Source: CAD feature listing. Evaluate the final solid. Frame: model axes, mm. A direction names the side the tool comes from. Round coordinates to 2 decimals unless told otherwise and drop trailing zeros. Order: outer loops, then holes, each group sorted by start corner. A loop starts at its lowest first (then second) coordinate and runs counter-clockwise, first axis right, second up. Notation, with made-up numbers: (73.5, -7) -> (77.5, -7) arc R18 cw to (77.5, 0) -> close; hole circle Ø3 at (-5.75, 24). An arc over 180 degrees is marked (long way). Answer as CSV lines item,"result". Start each with the question number.
(1) Section query C-C (z = 43). Output: boundary loops of the cut face in (x, y).
(2) Set-up query: faces 1 (the flat face through (17, 18, 5)), 2 (the flat face through (23.42, -21.22, 32.33)), 3 (the flat face through (0, 20, 5)), 4 (the flat face through (20, 0, 5)). Return all of +Z, -Z, +X, -X, +Y, -Y with unobstructed straight access to the full face (end or side cutting, diameter ignored); none if empty.
(3) Line query: line 1 along Y through (x, z) = (-15, 37); line 2 along X through (y, z) = (7.5, 8.5); line 3 along Z through (x, y) = (15, -24). Output: solid intervals per line, ascending. Write a range as from..to.
(4) Contact query for flat-ended pins moving along their axis: P1, Ø5, axis at x = 7, z = 4.5, coming from the +Y side; P2, Ø12, axis at y = -24.5, z = 8, coming from the +X side; P3, Ø12, axis at x = 25, z = 20, coming from the -Y side. Output: stop coordinate, or through.
(5) Section query A-A (z = 8.5). Output: boundary loops of the cut face in (x, y), plus the area to 3 significant figures.
(6) Section query B-B (z = 34.5). Output: boundary loops of the cut face in (x, y), plus the area to 3 significant figures.
(7) Pull-direction query (Z, two-part tool) for faces 5 (the flat face through (-21, -2, 10)), 6 (the flat face through (-17, -18, 5)), 7 (the flat face through (23.5, -10.2, 32.3)); classes: +Z half, -Z half, draft (parallel to the pull), parting line (faces both ways), or undercut.
```python
from build123d import *

# Parameters (mm, degrees)
F0_W      = 40
F0_H      = 40
F1_DEPTH  = 10
F2_SIZE   = 5
F3_W      = 50
F3_H      = 50
F4_DEPTH  = 10
F4_TAPER  = -20
F5_W      = 32.2794046853
F5_H      = 32.2794046853
F6_DEPTH  = 20
F8_DEPTH  = 25
F10_DEPTH = 3


with BuildPart() as f1:
    # F0 (on Top) → F1 (new body)
    with BuildSketch(Plane.XY):
        Rectangle(F0_W, F0_H)
    extrude(amount=F1_DEPTH)

    # F2
    f2_edges = [f1.edges().sort_by_distance(p)[0] for p in [
        (-20, -20, 5),
        (-20, 20, 5),
        (20, -20, 5),
        (20, 20, 5),
    ]]
    chamfer(f2_edges, length=F2_SIZE)

    # F3 (on face) → F4 (join)
    with BuildSketch(Plane.XY.offset(10)):
        Rectangle(F3_W, F3_H)
    extrude(amount=F4_DEPTH, taper=F4_TAPER)

    # F5 (on face) → F6 (join)
    with BuildSketch(Plane.XY.offset(20)):
        with Locations((-7.5, 2.5)):
            Rectangle(F5_W, F5_H)
    extrude(amount=F6_DEPTH)

    # F7 (on face) → F8 (join)
    with BuildSketch(Plane.XY.offset(20)):
        Polygon((20.2888493816, -26.6397023427), (26.6397023427, -15.6397023427), (20.2888493816, -4.6397023427), (7.5871434594, -4.6397023427), (1.2362904983, -15.6397023427), (7.5871434594, -26.6397023427), align=None)
    extrude(amount=F8_DEPTH)

    # F9 (on face) → F10 (join)
    with BuildSketch(Plane.XY.offset(45)):
        Polygon((23.1756007275, -31.6397023427), (32.4132050346, -15.6397023427), (23.1756007275, 0.3602976573), (4.7003921135, 0.3602976573), (-4.5372121936, -15.6397023427), (4.7003921135, -31.6397023427), align=None)
    extrude(amount=F10_DEPTH)


solid = f1.part
```
Answer block:
1,outline,"(1.24, -15.64) -> (7.59, -26.64) -> (20.29, -26.64) -> (26.64, -15.64) -> (20.29, -4.64) -> (7.59, -4.64) -> close"
2,face 1,"-Z, +X, +Y"
2,face 2,"+X, -Y"
2,face 3,"-Z, +X, -X, +Y"
2,face 4,"-Z, +X, +Y, -Y"
3,line 1,"-13.64..18.64"
3,line 2,"-20..20"
3,line 3,"10..48"
4,P1,"y = 20"
4,P2,"x = 26.46"
4,P3,"y = -28.64"
5,outline,"(-20, -15) -> (-15, -20) -> (15, -20) -> (20, -15) -> (20, 15) -> (15, 20) -> (-15, 20) -> (-20, 15) -> close"
5,area,"1,550 mm2"
6,outline,"(-23.64, -13.64) -> (2.39, -13.64) -> (1.24, -15.64) -> (7.59, -26.64) -> (20.29, -26.64) -> (26.64, -15.64) -> (20.29, -4.64) -> (8.64, -4.64) -> (8.64, 18.64) -> (-23.64, 18.64) -> close"
6,area,"1,430 mm2"
7,face 5,"-Z half"
7,face 6,"draft"
7,face 7,"undercut"
